Source: CAD feature listing. Evaluate the final solid. Frame: model axes, mm. A direction names the side the tool comes from. Give positions to 0.01 mm unless a question says otherwise; leave off trailing zeros. Loops run counter-clockwise (first coordinate to the right, second up) from the corner with the lowest first, then second, coordinate; pieces in that order, holes last. Notation, with made-up numbers: M 65.5,80 L 69.5,80 A33 ccw 69.5,111 Z; hole C -12,24.25 d6. An arc over 180 degrees is marked long. Put each result on its own line as item: value.
from build123d import *

# Parameters (mm, degrees)
SKETCH3_R           = 1.6
CUT_EXTRUDE1_DEPTH  = 10
SKETCH4_R           = 50
SKETCH4_R_2         = 40
BOSS_EXTRUDE1_DEPTH = 40


with BuildPart() as part:
    # Sketch1 → Revolve1 (revolve)
    with BuildSketch(Plane.XY, mode=Mode.PRIVATE) as revolve1_sk:
        Polygon((38, 0), (38, 9), (60, 9), (60, -9), (40.25, -9), (40.25, 0), align=None)
    revolve(revolve1_sk.sketch.rotate(Axis((0, 83.520836207, 0), (0, -1, 0)), 90), axis=Axis((0, 83.520836207, 0), (0, -1, 0)))

    # Sketch3 → Cut-Extrude1 (cut)
    with BuildSketch(Plane.XZ.offset(9)):
        with Locations(Location((0, 45.125, 0), (0, 0, 270))):
            Circle(SKETCH3_R)
        with Locations(Location((45.125, 0, 0), (0, 0, 270))):
            Circle(SKETCH3_R)
        with Locations(Location((0, -45.125, 0), (0, 0, 270))):
            Circle(SKETCH3_R)
        with Locations(Location((-45.125, 0, 0), (0, 0, 270))):
            Circle(SKETCH3_R)
    extrude(amount=-CUT_EXTRUDE1_DEPTH, mode=Mode.SUBTRACT)

    # Sketch4 → Boss-Extrude1 (add)
    with BuildSketch(Plane(origin=(0, 9, 0), x_dir=(1, 0, 0), z_dir=(0, 1, 0))):
        with Locations(Location((0, 0, 0), (0, 0, 270))):
            Circle(SKETCH4_R)
        with Locations(Location((0, 0, 0), (0, 0, 270))):
            Circle(SKETCH4_R_2, mode=Mode.SUBTRACT)
    extrude(amount=BOSS_EXTRUDE1_DEPTH)


solid = part.part
1. Draft query along Z for faces 4 (the flat face through (34, 49, -22)), 5 (the cylindrical face through (15.02, 28.72, 47.69)), 6 (the flat face through (-24, 0, 30)). Return one class per face: pulls with the +Z half, pulls with the -Z half, needs draft (parallel to the pull), parting line crosses it, or undercut.
Found:
face 4: needs draft
face 5: parting line crosses it
face 6: undercut
2. Contact query for flat-ended pins moving along their axis: P1, Ø12, axis at y = -2, z = -18.5, coming from the +X side; P2, Ø2, axis at x = 2.5, y = 13.5, coming from the -Z side; P3, Ø1.5, axis at x = 47.5, y = 9.5, coming from the +Z side. Output: stop coordinate, or through.
Found:
P1: x = 58.68
P2: z = -49.98
P3: z = 37.37
3. Section query C-C (y = 44). Output: boundary loops of the cut face in (x, z), plus the area to 3 significant figures.
Found:
outline: C 0,0 d100; hole C 0,0 d80
area: 2,830 mm^2
4. Material intervals for line 1 (X direction, y = -5, z = 0) (3 decimals); line 2 (X direction, y = 4.5, z = 0); line 3 (X direction, y = 25, z = 2), sorted ascending. Write a range as from..to.
Found:
line 1: -60..-46.725, -43.525..-40.25, 40.25..43.525, 46.725..60
line 2: -60..-38, 38..60
line 3: -49.96..-39.95, 39.95..49.96
5. Section query D-D (x = 0). Output: boundary loops of the cut face in (y, z) (3 decimals), plus the area to 3 significant figures.
Found:
outline: M -9,-60 L 9,-60 L 9,-50 L 49,-50 L 49,-40 L 9,-40 L 9,-38 L 0,-38 L 0,-40.25 L -9,-40.25 L -9,-43.525 L 1,-43.525 L 1,-46.725 L -9,-46.725 Z; M -9,40.25 L 0,40.25 L 0,38 L 9,38 L 9,40 L 49,40 L 49,50 L 9,50 L 9,60 L -9,60 L -9,46.725 L 1,46.725 L 1,43.525 L -9,43.525 Z
area: 1,490 mm^2
6. Section query B-B (x = 16.5). Output: boundary loops of the cut face in (y, z), plus the area to 3 significant figures.
Found:
outline: M -9,-57.69 L 9,-57.69 L 9,-47.2 L 49,-47.2 L 49,-36.44 L 9,-36.44 L 9,-34.23 L 0,-34.23 L 0,-36.71 L -9,-36.71 Z; M -9,36.71 L 0,36.71 L 0,34.23 L 9,34.23 L 9,36.44 L 49,36.44 L 49,47.2 L 9,47.2 L 9,57.69 L -9,57.69 Z
area: 1,660 mm^2
7. Access query for faces 1 (the flat face through (-45, 9, 23)), 2 (the cylindrical face through (-50.59, -0.13, 32.26)), 3 (the flat face through (0, 1, -45)). Directions: +Z, -Z, +X, -X, +Y, -Y. A direction counts if a zero-diameter tool reaches every point of the face in a straight line with its end or side. Return the directions, or none.
Found:
face 1: +Y
face 2: +Y, -Y
face 3: -Y
8. Section query A-A (z = 0). Output: boundary loops of the cut face in (x, y) (3 decimals).
Found:
outline: M -60,-9 L -46.725,-9 L -46.725,1 L -43.525,1 L -43.525,-9 L -40.25,-9 L -40.25,0 L -38,0 L -38,9 L -40,9 L -40,49 L -50,49 L -50,9 L -60,9 Z; M 38,0 L 40.25,0 L 40.25,-9 L 43.525,-9 L 43.525,1 L 46.725,1 L 46.725,-9 L 60,-9 L 60,9 L 50,9 L 50,49 L 40,49 L 40,9 L 38,9 Z
